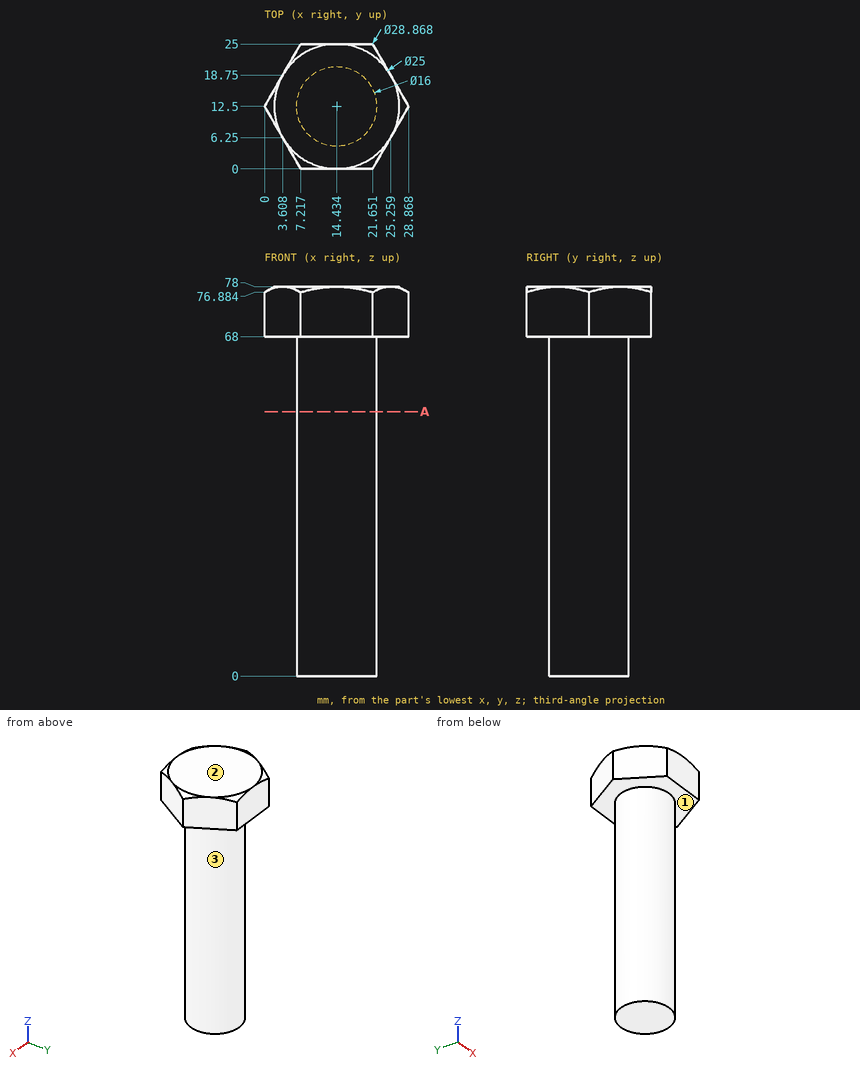
Job drawing, mm, ordinate dimensions from the low corner. One solid piece. Coordinates: 2 decimals unless noted, no trailing zeros. Order: outer loops, then holes, each group sorted by start corner. A loop starts at its lowest first (then second) coordinate and runs counter-clockwise, first axis right, second up. Notation, with made-up numbers: (47, 38) -> (59, 38) arc R25 ccw to (59, 58) -> close; hole circle Ø4 at (37.5, 35.25). An arc over 180 degrees is marked (long way). Answer in a Markdown table with one row per item. Add a question column.
Q1. Band-saw the part on A-A, the plane z = 53. List the corners of the cut face in (x, y).
Q2. Drop flat-ended pins along their axis: pin 1 (10 mm diameter, centred on x = 14.5, z = 52.5, fed in from +Y); pin 2 (2 mm diameter, centred on y = 6, z = 29, fed in from +X) (1 decimal); pin 3 (10 mm diameter, centred on y = 20, z = 15.5, fed in from -X) (1 decimal). Give the stop position or say it passes through.
Q3. Mould opens along Z. For the marked faces 1, 2 and 3 say: +Z half, -Z half, draft (parallel to the pull), parting line (faces both ways), or undercut.
Q4. Wall check: line 1 along Z through (x, y) = (22.5, 13.25); line 2 along X through (y, z) = (10, 28.5) (1 decimal); line 3 along Y through (x, z) = (14, 21.5). Give the ranges that are in metal, low to high. Write a range as [from, to].
Answers follow:
| question | item | result |
|---|---|---|
| 1 | outline | circle Ø16 at (14.43, 12.5) |
| 2 | pin 1 | y = 20.5 |
| 2 | pin 2 | x = 20.2 |
| 2 | pin 3 | x = 6.8 |
| 3 | face 1 | -Z half |
| 3 | face 2 | +Z half |
| 3 | face 3 | draft |
| 4 | line 1 | [68, 78] |
| 4 | line 2 | [6.8, 22] |
| 4 | line 3 | [4.51, 20.49] |
